Geometry check sheet. Reference: the model listing, model coordinates, mm. A direction names the side the tool comes from. Coordinates: 2 decimals unless noted, no trailing zeros. Write each loop counter-clockwise with the first axis right and the second up, starting at its lowest first coordinate (ties: lowest second). Pieces come first, ordered by that corner, then holes.
from build123d import *

# Parameters (mm, degrees)
SKETCH_2_R                    = 75
EXTRUDE_1_DEPTH               = 10
SKETCH_3_R                    = 60
EXTRUDE_3_DEPTH               = 34.3
SHELL_2_T                     = -6
CUT_EXTRUDE_START             = -25
CUT_EXTRUDE_2_DEPTH           = 25
EXTRUDE_START                 = -15
EXTRUDE_4_DEPTH               = 15
HOLE_WIZARD_M3_5_1_AT_2_COUNT = 2
HOLE_WIZARD_M3_5_1_AT_2_PITCH = 60.104076401
HOLE_WIZARD_M3_5_1_AT_3_COUNT = 2
HOLE_WIZARD_M3_5_1_AT_3_PITCH = 85
HOLE_WIZARD_M3_5_1_AT_4_COUNT = 2
HOLE_WIZARD_M3_5_1_AT_4_PITCH = 60.104076401
PATTERN_CIRCULAR_1_COUNT      = 4
PATTERN_CIRCULAR_1_ANGLE      = 135


with BuildPart() as part:
    # 草图2 → 凸台-拉伸1 (new body)
    with BuildSketch(Plane.XY):
        with Locations((-40.151148837, 28.730605226)):
            Circle(SKETCH_2_R)
    extrude(amount=EXTRUDE_1_DEPTH)

    # 草图3 → 凸台-拉伸3 (add)
    with BuildSketch(Plane(origin=(0, 0, 0), x_dir=(-1, 0, 0), z_dir=(0, 0, -1))):
        with Locations((40.151148837, 28.730605226)):
            Circle(SKETCH_3_R)
    extrude(amount=EXTRUDE_3_DEPTH)

    # 抽壳2
    shell_2_openings = [part.faces().sort_by_distance(p)[0] for p in [
        (-40.151148837, 28.730605226, -34.3),
    ]]
    offset(amount=SHELL_2_T, openings=shell_2_openings, kind=Kind.INTERSECTION)

    # 草图5 → 切除-拉伸2 (cut)
    with BuildSketch(Plane(origin=(0, 0, -34.3), x_dir=(-1, 0, 0), z_dir=(0, 0, -1)).offset(CUT_EXTRUDE_START)):
        with BuildLine():
            ThreePointArc((75.263111693, 77.38397165), (40.151148837, 88.730605226), (5.039185981, 77.38397165))
            Line((5.039185981, 77.38397165), (5.039185981, 69.756817145))
            ThreePointArc((5.039185981, 69.756817145), (40.151148837, 82.730605226), (75.263111693, 69.756817145))
            Line((75.263111693, 69.756817145), (75.263111693, 77.38397165))
        make_face()
        with BuildLine():
            Line((5.039185981, -12.295606692), (5.039185981, -19.922761198))
            ThreePointArc((5.039185981, -19.922761198), (40.567011683, -31.267953574), (75.934159557, -19.43137297))
            Line((75.934159557, -19.43137297), (75.934159557, -11.711651681))
            ThreePointArc((75.934159557, -11.711651681), (40.595926503, -25.26756301), (5.039185981, -12.295606692))
        make_face()
    extrude(amount=CUT_EXTRUDE_2_DEPTH, mode=Mode.SUBTRACT)

    # 草图6 → 凸台-拉伸4 (add)
    with BuildSketch(Plane(origin=(0, 0, -34.3), x_dir=(-1, 0, 0), z_dir=(0, 0, -1)).offset(EXTRUDE_START)):
        with BuildLine():
            Line((5.039185981, 77.38397165), (5.039185981, 69.756817145))
            ThreePointArc((5.039185981, 69.756817145), (40.151148837, 82.730605226), (75.263111693, 69.756817145))
            Line((75.263111693, 69.756817145), (75.263111693, 77.38397165))
            ThreePointArc((75.263111693, 77.38397165), (40.151148837, 88.730605226), (5.039185981, 77.38397165))
        make_face()
        with BuildLine():
            Line((75.934159557, -11.711651681), (75.934159557, -19.43137297))
            ThreePointArc((75.934159557, -19.43137297), (40.567011683, -31.267953574), (5.039185981, -19.922761198))
            Line((5.039185981, -19.922761198), (5.039185981, -12.295606692))
            ThreePointArc((5.039185981, -12.295606692), (40.595926503, -25.26756301), (75.934159557, -11.711651681))
        make_face()
    extrude(amount=EXTRUDE_4_DEPTH)

    # 草图10 → M3.5 螺纹孔1 (revolve, cut)
    with BuildSketch(Plane(origin=(2.348851163, 28.730605226, 4), x_dir=(0, 1, 0), z_dir=(1, 0, 0))):
        Polygon((0, 0), (0, 5.871247898), (1.45, 5), (1.45, 0.325), (1.775, 0), align=None)
    hole_wizard_m3_5_1 = revolve(axis=Axis((2.348851163, 28.730605226, -2.35), (0, 0, 1)), mode=Mode.SUBTRACT)

    # M3.5 螺纹孔1 at 2: M3.5 螺纹孔1 ×2
    with Locations(*[Vector(-0.7071067811865475, 0.7071067811865476, 0) * (i * HOLE_WIZARD_M3_5_1_AT_2_PITCH) for i in range(1, HOLE_WIZARD_M3_5_1_AT_2_COUNT)]):
        add(hole_wizard_m3_5_1, mode=Mode.SUBTRACT)

    # M3.5 螺纹孔1 at 3: M3.5 螺纹孔1 ×2
    with Locations(*[(-i * HOLE_WIZARD_M3_5_1_AT_3_PITCH, 0, 0) for i in range(1, HOLE_WIZARD_M3_5_1_AT_3_COUNT)]):
        add(hole_wizard_m3_5_1, mode=Mode.SUBTRACT)

    # M3.5 螺纹孔1 at 4: M3.5 螺纹孔1 ×2
    with Locations(*[Vector(-0.7071067811865476, -0.7071067811865476, 0) * (i * HOLE_WIZARD_M3_5_1_AT_4_PITCH) for i in range(1, HOLE_WIZARD_M3_5_1_AT_4_COUNT)]):
        add(hole_wizard_m3_5_1, mode=Mode.SUBTRACT)

    # 阵列(圆周)1: M3.5 螺纹孔1 ×4 about axis
    pattern_circular_1_axis = Axis((-40.151148837, 28.730605226, 0), (0, 0, -1))
    for i in range(1, PATTERN_CIRCULAR_1_COUNT):
        add(hole_wizard_m3_5_1.rotate(pattern_circular_1_axis, i * PATTERN_CIRCULAR_1_ANGLE / (PATTERN_CIRCULAR_1_COUNT - 1)), mode=Mode.SUBTRACT)

    # 阵列(圆周)1 copy 1 sketch → 阵列(圆周)1 copy 1 (revolve, cut)
    with BuildSketch(Plane(origin=(-10.099110636, 58.782643427, 4), x_dir=(0.7071067811865487, 0.7071067811865464, 0), z_dir=(0.7071067811865464, -0.7071067811865487, 0))):
        Polygon((0, 0), (0, 5.871247898), (1.45, 5), (1.45, 0.325), (1.775, 0), align=None)
    revolve(axis=Axis((-10.099110636, 58.782643427, -2.35), (0, 0, 1)), mode=Mode.SUBTRACT)

    # 阵列(圆周)1 copy 2 sketch → 阵列(圆周)1 copy 2 (revolve, cut)
    with BuildSketch(Plane(origin=(2.348851163, 28.730605226, 4), x_dir=(1, 0, 0), z_dir=(0, -1, 0))):
        Polygon((0, 0), (0, 5.871247898), (1.45, 5), (1.45, 0.325), (1.775, 0), align=None)
    revolve(axis=Axis((2.348851163, 28.730605226, -2.35), (0, 0, 1)), mode=Mode.SUBTRACT)

    # 阵列(圆周)1 copy 3 sketch → 阵列(圆周)1 copy 3 (revolve, cut)
    with BuildSketch(Plane(origin=(-10.099110636, -1.321432974, 4), x_dir=(0.7071067811865441, -0.7071067811865509, 0), z_dir=(-0.7071067811865509, -0.7071067811865441, 0))):
        Polygon((0, 0), (0, 5.871247898), (1.45, 5), (1.45, 0.325), (1.775, 0), align=None)
    revolve(axis=Axis((-10.099110636, -1.321432974, -2.35), (0, 0, 1)), mode=Mode.SUBTRACT)

    # 阵列(圆周)1 copy 4 sketch → 阵列(圆周)1 copy 4 (revolve, cut)
    with BuildSketch(Plane(origin=(-70.203187037, 58.782643427, 4), x_dir=(0.7071067811865487, 0.7071067811865464, 0), z_dir=(0.7071067811865464, -0.7071067811865487, 0))):
        Polygon((0, 0), (0, 5.871247898), (1.45, 5), (1.45, 0.325), (1.775, 0), align=None)
    revolve(axis=Axis((-70.203187037, 58.782643427, -2.35), (0, 0, 1)), mode=Mode.SUBTRACT)

    # 阵列(圆周)1 copy 5 sketch → 阵列(圆周)1 copy 5 (revolve, cut)
    with BuildSketch(Plane(origin=(-40.151148837, 71.230605226, 4), x_dir=(1, 0, 0), z_dir=(0, -1, 0))):
        Polygon((0, 0), (0, 5.871247898), (1.45, 5), (1.45, 0.325), (1.775, 0), align=None)
    revolve(axis=Axis((-40.151148837, 71.230605226, -2.35), (0, 0, 1)), mode=Mode.SUBTRACT)

    # 阵列(圆周)1 copy 6 sketch → 阵列(圆周)1 copy 6 (revolve, cut)
    with BuildSketch(Plane(origin=(-10.099110636, 58.782643427, 4), x_dir=(0.7071067811865441, -0.7071067811865509, 0), z_dir=(-0.7071067811865509, -0.7071067811865441, 0))):
        Polygon((0, 0), (0, 5.871247898), (1.45, 5), (1.45, 0.325), (1.775, 0), align=None)
    revolve(axis=Axis((-10.099110636, 58.782643427, -2.35), (0, 0, 1)), mode=Mode.SUBTRACT)

    # 阵列(圆周)1 copy 7 sketch → 阵列(圆周)1 copy 7 (revolve, cut)
    with BuildSketch(Plane(origin=(-70.203187037, -1.321432974, 4), x_dir=(0.7071067811865487, 0.7071067811865464, 0), z_dir=(0.7071067811865464, -0.7071067811865487, 0))):
        Polygon((0, 0), (0, 5.871247898), (1.45, 5), (1.45, 0.325), (1.775, 0), align=None)
    revolve(axis=Axis((-70.203187037, -1.321432974, -2.35), (0, 0, 1)), mode=Mode.SUBTRACT)

    # 阵列(圆周)1 copy 8 sketch → 阵列(圆周)1 copy 8 (revolve, cut)
    with BuildSketch(Plane(origin=(-82.651148837, 28.730605226, 4), x_dir=(1, 0, 0), z_dir=(0, -1, 0))):
        Polygon((0, 0), (0, 5.871247898), (1.45, 5), (1.45, 0.325), (1.775, 0), align=None)
    revolve(axis=Axis((-82.651148837, 28.730605226, -2.35), (0, 0, 1)), mode=Mode.SUBTRACT)

    # 阵列(圆周)1 copy 9 sketch → 阵列(圆周)1 copy 9 (revolve, cut)
    with BuildSketch(Plane(origin=(-70.203187037, 58.782643427, 4), x_dir=(0.7071067811865441, -0.7071067811865509, 0), z_dir=(-0.7071067811865509, -0.7071067811865441, 0))):
        Polygon((0, 0), (0, 5.871247898), (1.45, 5), (1.45, 0.325), (1.775, 0), align=None)
    revolve(axis=Axis((-70.203187037, 58.782643427, -2.35), (0, 0, 1)), mode=Mode.SUBTRACT)


solid = part.part
1. Draft check along Y on faces 5 (the cylindrical face through (31.385, 51.259, 4.93)), 6 (the flat face through (-41, 29, 4)), 7 (the flat face through (13.5, 37.9, -34.3)). Enter one of: released by +Y, released by -Y, zero draft, split by the parting line, or undercut.
Computed values:
face 5: split by the parting line
face 6: undercut
face 7: zero draft
2. Sectioned sample at D-D, the plane x = -97. Record the boundary of the cut face in (y, z).
Computed values:
outline: (-20.19, 0) - (9.54, 0) - (9.54, -34.3) - (47.92, -34.3) - (47.92, 0) - (77.65, 0) - (77.65, 10) - (-20.19, 10) - close
3. Gauge pin test, flat ends, axial feed: pin 1 Ø6 at (y, z) = (65, -6) entering from +X; pin 2 Ø2.5 at (y, z) = (-16.5, -12.5) entering from -X; pin 3 Ø5 at (x, z) = (-76.5, -4.5) entering from -Y. Record the tip position at first contact, or that the pin passes through.
Computed values:
pin 1: stops at x = 9.78
pin 2: stops at x = -80.96
pin 3: stops at y = -20.81
4. Access from +Z, -Z, +X, -X, +Y, -Y to the whole of each face (thin tool, end or side, straight path). Record for faces 1 (the flat face through (-41, 30, 10)), 2 (the flat face through (-75.934, -16, -14)), 3 (the flat face through (-74, 79, 0)), 4 (the flat face through (-5.039, 74, -14)).
Computed values:
face 1: +Z, +X, -X, +Y, -Y
face 2: -Y
face 3: -Z
face 4: +Y, -Y
5. Sectioned sample at A-A, the plane z = -14. Record the boundary of the cut face in (x, y).
Computed values:
outline: (-75.93, -19.43) - (-75.93, -11.71) arc R54 cw to (-75.26, 69.76) - (-75.26, 77.38) arc R60 ccw to start; (-5.04, -19.92) arc R60 ccw to (-5.04, 77.38) - (-5.04, 69.76) arc R54 cw to (-5.04, -12.3) - close
6. Thickness scan on line 1 along Z through (x, y) = (-27, 83.5); line 2 along Y through (x, z) = (-10, 8); line 3 along Z through (x, y) = (-75.5, 17.5). Record the ranges inside material, lowest first.
Computed values:
line 1: z = -34.3 to -19.3, -9.3 to 10
line 2: y = -39.94 to -2.77, 0.13 to 57.34, 60.23 to 97.4
line 3: z = 4 to 10
7. Sectioned sample at C-C, the plane y = -8. Record the boundary of the cut face in (x, z), and give its area (3 significant figures).
Computed values:
outline: (-105.54, 0) - (-87.59, 0) - (-87.59, -34.3) - (-79.73, -34.3) - (-79.73, 4) - (-0.57, 4) - (-0.57, -34.3) - (7.29, -34.3) - (7.29, 0) - (25.24, 0) - (25.24, 10) - (-105.54, 10) - close
area: 1,530 mm2
8. Sectioned sample at B-B, the plane x = -26. Record the boundary of the cut face in (y, z).
Computed values:
outline: (-44.92, 0) - (-29.58, 0) - (-29.58, -9.3) - (-23.38, -9.3) - (-23.38, 4) - (80.84, 4) - (80.84, -9.3) - (87.04, -9.3) - (87.04, 0) - (102.38, 0) - (102.38, 10) - (-44.92, 10) - close; (-29.58, -34.3) - (-23.38, -34.3) - (-23.38, -19.3) - (-29.58, -19.3) - close; (80.84, -34.3) - (87.04, -34.3) - (87.04, -19.3) - (80.84, -19.3) - close
